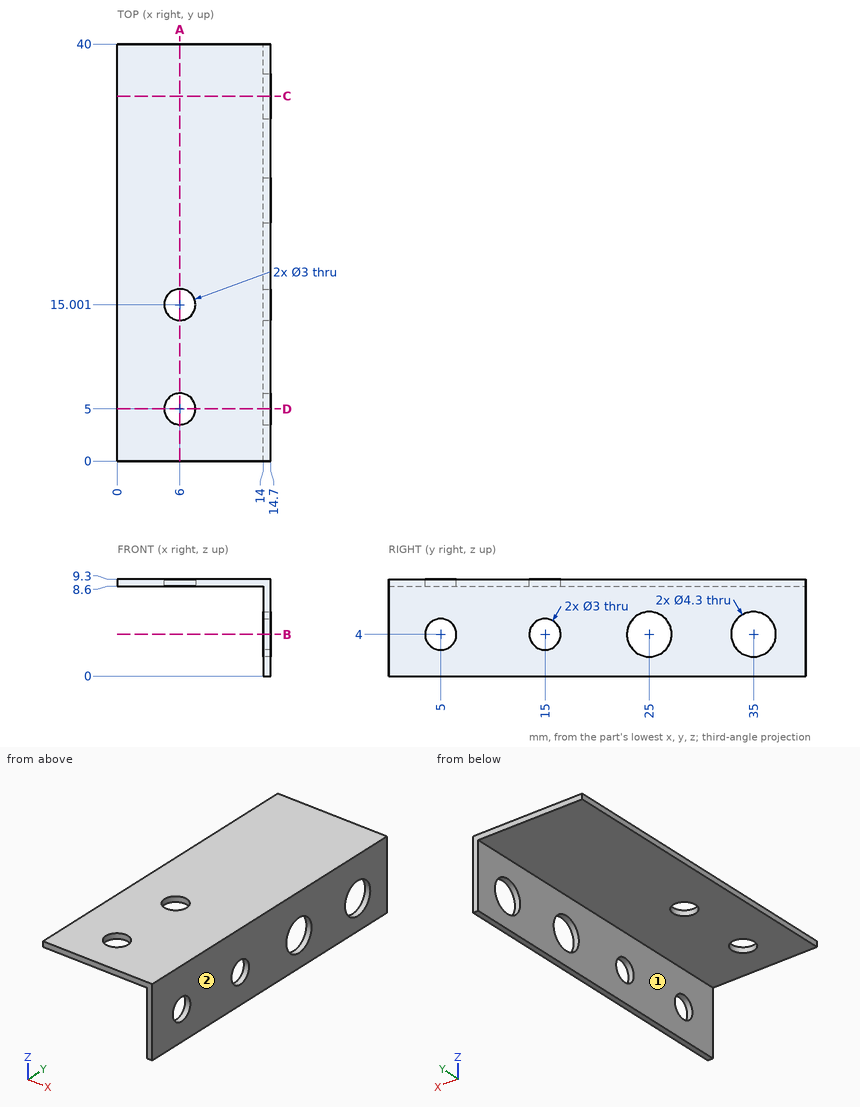
The drawing under review shows one solid part. Ordinate dimensions are in mm from its lowest x, y, z. A direction names the side the tool comes from. Round coordinates to 2 decimals unless told otherwise and drop trailing zeros. Order: outer loops, then holes, each group sorted by start corner. A loop starts at its lowest first (then second) coordinate and runs counter-clockwise, first axis right, second up. Notation, with made-up numbers: (23.25, 18) - (34.25, 18) arc R25 cw to (34.25, 35) - close; hole circle Ø11 at (55, 11). An arc over 180 degrees is marked (long way). Return JSON: item names as keys, results as strings.
Q1. Wall thickness on L1, parallel to Y at x = 6, z = 9.15; L2, parallel to Y at x = 14.2, z = 4; L3, parallel to X at y = 13, z = 7.25: over which ranges is each line inside the solid? List them lowest first. Write a range as [from, to].
Computed values:
{"L1": "y = [0, 3.5], [6.5, 13.5], [16.5, 40]", "L2": "y = [0, 3.5], [6.5, 13.5], [16.5, 22.85], [27.15, 32.85], [37.15, 40]", "L3": "x = [14, 14.7]"}
Q2. Machinability: for the marked faces 1 and 2, which of the approach directions +Z, -Z, +X, -X, +Y, -Y give a long, thin tool a straight path to every point of the face, cutting with its end or side? Answer none if there is none.
Computed values:
{"face 1": "-Z, -X, +Y, -Y", "face 2": "+Z, -Z, +X, +Y, -Y"}
Q3. For pin 1 Ø5.5 at (y, z) = (35, 4) entering from +X; pin 2 Ø7 at (x, y) = (4, 22) entering from -Z; pin 3 Ø5 at (y, z) = (15, 4) entering from -X, all flat-tipped, find the tip position at first contact; note any pin that passes through.
Computed values:
{"pin 1": "stops at x = 14.7", "pin 2": "stops at z = 8.6", "pin 3": "stops at x = 14"}
Q4. Consider section A-A on x = 6. Write out the cut boundary in (y, z).
Computed values:
{"outline": "(0, 8.6) - (3.5, 8.6) - (3.5, 9.3) - (0, 9.3) - close; (6.5, 8.6) - (13.5, 8.6) - (13.5, 9.3) - (6.5, 9.3) - close; (16.5, 8.6) - (40, 8.6) - (40, 9.3) - (16.5, 9.3) - close"}
Q5. Consider section D-D on y = 5. Write out the cut boundary in (x, z), plus the area to 3 significant figures.
Computed values:
{"outline": "(0, 8.6) - (4.5, 8.6) - (4.5, 9.3) - (0, 9.3) - close; (7.5, 8.6) - (14, 8.6) - (14, 5.5) - (14.7, 5.5) - (14.7, 9.3) - (7.5, 9.3) - close; (14, 0) - (14.7, 0) - (14.7, 2.5) - (14, 2.5) - close", "area": "12.1 mm2"}
Q6. Consider section C-C on y = 35. Write out the cut boundary in (x, z).
Computed values:
{"outline": "(0, 8.6) - (14, 8.6) - (14, 6.15) - (14.7, 6.15) - (14.7, 9.3) - (0, 9.3) - close; (14, 0) - (14.7, 0) - (14.7, 1.85) - (14, 1.85) - close"}
Q7. Consider section B-B on z = 4. Write out the cut boundary in (x, y), plus the area to 3 significant figures.
Computed values:
{"outline": "(14, 0) - (14.7, 0) - (14.7, 3.5) - (14, 3.5) - close; (14, 6.5) - (14.7, 6.5) - (14.7, 13.5) - (14, 13.5) - close; (14, 16.5) - (14.7, 16.5) - (14.7, 22.85) - (14, 22.85) - close; (14, 27.15) - (14.7, 27.15) - (14.7, 32.85) - (14, 32.85) - close; (14, 37.15) - (14.7, 37.15) - (14.7, 40) - (14, 40) - close", "area": "17.8 mm2"}
